```python
from build123d import *

# Parameters (mm, degrees)
BOSS_EXTRUDE1_DEPTH   = 15
SKETCH1_R             = 50
SKETCH1_R_2           = 5
SKETCH1_R_3           = 20
BOSS_EXTRUDE1_2_DEPTH = 15
BOSS_EXTRUDE2_DEPTH   = 9


with BuildPart() as part:
    # Sketch1 → Boss-Extrude1 (new, symmetric)
    with BuildSketch(Plane(origin=(0, 0, 0), x_dir=(1, 0, 0), z_dir=(0, 1, 0))):
        with BuildLine():
            ThreePointArc((30, 51.961524227), (0, 60), (-30, 51.961524227))
            ThreePointArc((-30, 51.961524227), (-57.320508076, 59.282032303), (-50, 86.602540378))
            ThreePointArc((-50, 86.602540378), (0, 100), (50, 86.602540378))
            ThreePointArc((50, 86.602540378), (57.320508076, 59.282032303), (30, 51.961524227))
        make_face()
        with BuildLine():
            ThreePointArc((-45, 77.942286341), (-48.660254038, 64.282032303), (-35, 60.621778265))
            ThreePointArc((-35, 60.621778265), (0, 70), (35, 60.621778265))
            ThreePointArc((35, 60.621778265), (48.660254038, 64.282032303), (45, 77.942286341))
            ThreePointArc((45, 77.942286341), (0, 90), (-45, 77.942286341))
        make_face(mode=Mode.SUBTRACT)
    extrude(amount=BOSS_EXTRUDE1_DEPTH, both=True)



with BuildPart() as body_2:
    # Sketch1 → Boss-Extrude1 2 (new, symmetric)
    with BuildSketch(Plane(origin=(0, 0, 0), x_dir=(1, 0, 0), z_dir=(0, 1, 0))):
        with Locations(Location((0, 0, 0), (0, 0, 270))):
            Circle(SKETCH1_R)
        with Locations(Location((17.5, 30.310889132, 0), (0, 0, 270))):
            Circle(SKETCH1_R_2, mode=Mode.SUBTRACT)
        with Locations(Location((-17.5, 30.310889132, 0), (0, 0, 270))):
            Circle(SKETCH1_R_2, mode=Mode.SUBTRACT)
        with Locations(Location((-35, 0, 0), (0, 0, 270))):
            Circle(SKETCH1_R_2, mode=Mode.SUBTRACT)
        with Locations(Location((-17.5, -30.310889132, 0), (0, 0, 270))):
            Circle(SKETCH1_R_2, mode=Mode.SUBTRACT)
        with Locations(Location((17.5, -30.310889132, 0), (0, 0, 270))):
            Circle(SKETCH1_R_2, mode=Mode.SUBTRACT)
        with Locations(Location((35, 0, 0), (0, 0, 270))):
            Circle(SKETCH1_R_2, mode=Mode.SUBTRACT)
        with Locations(Location((0, 0, 0), (0, 0, 270))):
            Circle(SKETCH1_R_3, mode=Mode.SUBTRACT)
    extrude(amount=BOSS_EXTRUDE1_2_DEPTH, both=True)


with BuildPart() as part_1:
    add(part.part)

    add(body_2.part)  # Boss-Extrude2 merges body 2
    # Sketch1_3 → Boss-Extrude2 (add, symmetric)
    with BuildSketch(Plane(origin=(0, 0, 0), x_dir=(1, 0, 0), z_dir=(0, 1, 0))):
        with BuildLine():
            ThreePointArc((-37.490169455, 33.08303484), (0, 50), (37.490169455, 33.08303484))
            ThreePointArc((37.490169455, 33.08303484), (35.561850492, 43.037885637), (43.325468897, 49.56043864))
            ThreePointArc((43.325468897, 49.56043864), (36.453361541, 49.599010288), (30, 51.961524227))
            ThreePointArc((30, 51.961524227), (0, 60), (-30, 51.961524227))
            ThreePointArc((-30, 51.961524227), (-36.453361541, 49.599010288), (-43.325468897, 49.56043864))
            ThreePointArc((-43.325468897, 49.56043864), (-35.561850492, 43.037885637), (-37.490169455, 33.08303484))
        make_face()
    extrude(amount=BOSS_EXTRUDE2_DEPTH, both=True)


solid = part_1.part
```
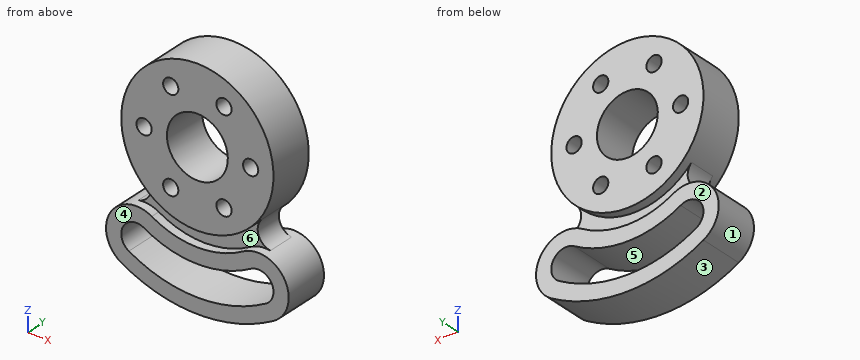
Design review of the part built by this model. Coordinates are the model's own, in mm. Face numbers are marked on the shaded views. A direction names the side the tool comes from. Give positions to 0.01 mm unless a question says otherwise; leave off trailing zeros. Order: outer loops, then holes, each group sorted by start corner. A loop starts at its lowest first (then second) coordinate and runs counter-clockwise, first axis right, second up. Notation, with made-up numbers: (7.25, 3) - (64.25, 3) arc R26 ccw to (64.25, 35) - close; hole circle Ø7 at (-8, 66). An arc over 180 degrees is marked (long way). Use a Markdown table: item, result. Add a question column.
(1) Wall thickness on probe 1 along X at (y, z) = (-2, 0); probe 2 along X at (y, z) = (-3.25, 32.5); probe 3 along Z at (x, y) = (-33, -7.5): over which ranges is each line inside the solid? List them lowest first. Write a range as [from, to].
(2) Mouldability with a two-part tool opening along Z and no side actions: class the marked faces 1, 2 and 3 as +Z half, -Z half, draft (parallel to the pull), parting line (faces both ways), or undercut.
(3) Machinability: for the marked faces 4, 5 and 6, which of the approach directions +Z, -Z, +X, -X, +Y, -Y give a long, thin tool a straight path to every point of the face, cutting with its end or side? Answer none if there is none.
(4) Add section D-D on x = -32. Give the boundary of the cut face in (y, z), then the cut area to 3 significant figures.
(5) Add section A-A on z = 0. Give the boundary of the cut face in (x, y), then the cut area to 3 significant figures.
(6) Add section C-C on z = 27.5. Give the boundary of the cut face in (x, y), then the cut area to 3 significant figures.
(7) Add section B-B on x = 17.5. Give the boundary of the cut face in (y, z), then the cut area to 3 significant figures.
(8) Clearance check with flat-ended pins moving along their axes: P1, Ø8, axis at x = 35, z = 0, coming from the -Y side; P2, Ø5, axis at x = -35, y = 6.5, coming from the +Z side; P3, Ø2, axis at y = 0.5, z = 27, coming from the +X side; P4, Ø5, axis at y = 7.5, z = -52.5, coming from the -X side. State where each tip first meets the part, or that it passes through.
Report:
| question | item | result |
|---|---|---|
| 1 | probe 1 | x = [-50, -40], [-30, -20], [20, 30], [40, 50] |
| 1 | probe 2 | x = [-38, -22], [-13, 13], [22, 38] |
| 1 | probe 3 | z = [-94.4, -83.73], [-61.73, -4.58], [4.58, 37.56] |
| 2 | face 1 | undercut |
| 2 | face 2 | draft |
| 2 | face 3 | -Z half |
| 3 | face 4 | +Z, -Z, +X, -X, -Y |
| 3 | face 5 | +Y, -Y |
| 3 | face 6 | -Y |
| 4 | outline | (-15, -94.74) - (15, -94.74) - (15, -84.12) - (-15, -84.12) - close; (-15, -62.26) - (15, -62.26) - (15, -50.95) - (9, -50.95) - (9, -38.42) - (15, -38.42) - (15, -4) - (-15, -4) - (-15, -38.42) - (-9, -38.42) - (-9, -50.95) - (-15, -50.95) - close; (-15, 4) - (15, 4) - (15, 38.42) - (-15, 38.42) - close |
| 4 | area | 2,950 mm² |
| 5 | outline | (-50, -15) - (-40, -15) - (-40, 15) - (-50, 15) - close; (-30, -15) - (-20, -15) - (-20, 15) - (-30, 15) - close; (20, -15) - (30, -15) - (30, 15) - (20, 15) - close; (40, -15) - (50, -15) - (50, 15) - (40, 15) - close |
| 5 | area | 1,200 mm² |
| 6 | outline | (-41.76, -15) - (-21.64, -15) - (-21.64, 15) - (-41.76, 15) - close; (-13.36, -15) - (13.36, -15) - (13.36, 15) - (-13.36, 15) - close; (21.64, -15) - (41.76, -15) - (41.76, 15) - (21.64, 15) - close |
| 6 | area | 2,010 mm² |
| 7 | outline | (-15, -98.46) - (15, -98.46) - (15, -88.28) - (-15, -88.28) - close; (-15, -67.78) - (15, -67.78) - (15, -57.39) - (9, -57.39) - (9, -46.84) - (15, -46.84) - (15, -35.31) - (-15, -35.31) - (-15, -46.84) - (-9, -46.84) - (-9, -57.39) - (-15, -57.39) - close; (-15, -25.31) - (15, -25.31) - (15, -9.68) - (-15, -9.68) - close; (-15, 9.68) - (15, 9.68) - (15, 25.31) - (-15, 25.31) - close; (-15, 35.31) - (15, 35.31) - (15, 46.84) - (-15, 46.84) - close |
| 7 | area | 2,440 mm² |
| 8 | P1 | passes through |
| 8 | P2 | stops at z = 38 |
| 8 | P3 | stops at x = 42.71 |
| 8 | P4 | stops at x = -54 |
